Study the drawing (mm; zero at the part's minimum x, y, z) and answer. A direction names the side the tool comes from. Round coordinates to 2 decimals unless told otherwise and drop trailing zeros. Write each loop counter-clockwise with the first axis right and the second up, starting at its lowest first coordinate (ties: lowest second). Pieces come first, ordered by that corner, then holes. Notation, with made-up numbers: (-12, 81.5) - (30, 81.5) arc R23 cw to (30, 106.5) - close; hole circle Ø11 at (15, 2). An arc over 180 degrees is marked (long way). Return JSON: item names as keys, results as strings. Group by question number.
(1) Section A-A, the plane y = 2.5 is taken. Write down the section's boundary in (x, z), then the cut area to 3 significant figures.
(2) Which of the six approach directions +Z, -Z, +X, -X, +Y, -Y give full straight-line access (tool end or side, diameter ignored) to the marked faces 1, 2, 3 and 4?
(3) Each of these flat-tipped pins is pushed along its axis until it touches: pin 1 (1.2 mm diameter, centred on x = 4.5, z = 2, fed in from +Y); pin 2 (3.5 mm diameter, centred on x = 7.5, y = 8.5, fed in from -Z); pin 3 (3.5 mm diameter, centred on x = 9, z = 19, fed in from +Y); pin 4 (1.3 mm diameter, centred on x = 6, z = 13.5, fed in from +Y). Where does it stop, or does it pass through?
(4) Section D-D, the plane y = 28.5 is taken. Write down the section's boundary in (x, z).
(5) Section C-C, the plane x = 4.25 is taken. Write down the section's boundary in (y, z), then the cut area to 3 significant figures.
(6) Find the intervals of material crossed by line 1 along Y through (x, z) = (7, 2); line 2 along Z through (x, y) = (1, 17.5); line 3 along Y through (x, z) = (3.5, 25.5), in increasing order. Write a range as [from, to].
(7) Section B-B, the plane z = 23.5 is taken. Write down the section's boundary in (x, y).
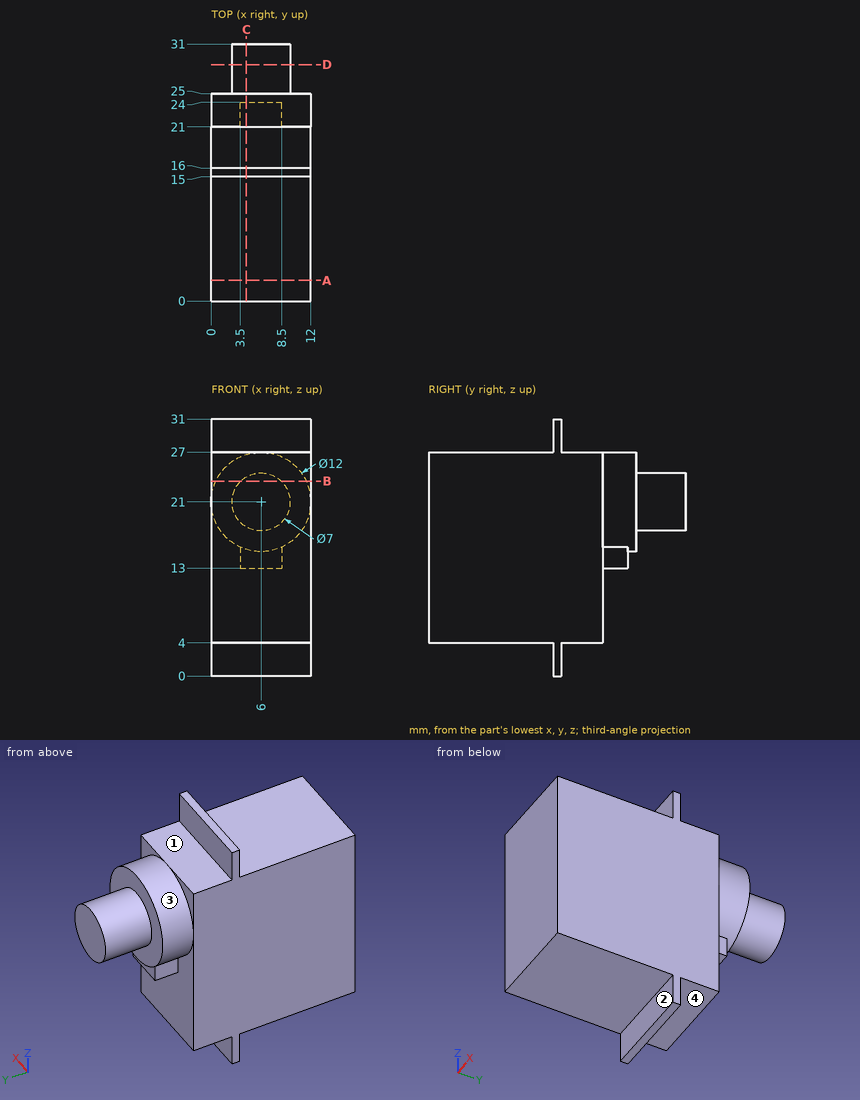
Working result:
{
 "1": {"outline": "(0, 4) - (12, 4) - (12, 27) - (0, 27) - close", "area": "276 mm^2"},
 "2": {"face 1": "+Z, +X, -X, +Y", "face 2": "-Z, +X, -X, -Y", "face 3": "+Y", "face 4": "-Z, +X, -X, +Y"},
 "3": {"pin 1": "stops at y = 16", "pin 2": "stops at z = 4", "pin 3": "stops at y = 31", "pin 4": "stops at y = 24"},
 "4": {"outline": "circle Ø7 at (6, 21)"},
 "5": {"outline": "(0, 4) - (15, 4) - (15, 0) - (16, 0) - (16, 4) - (21, 4) - (21, 13) - (24, 13) - (24, 15.26) - (25, 15.26) - (25, 17.97) - (31, 17.97) - (31, 24.03) - (25, 24.03) - (25, 26.74) - (21, 26.74) - (21, 27) - (16, 27) - (16, 31) - (15, 31) - (15, 27) - (0, 27) - close", "area": "580 mm^2"},
 "6": {"line 1": "y = [15, 16]", "line 2": "z = [4, 27]", "line 3": "y = [0, 25]"},
 "7": {"outline": "(0, 0) - (12, 0) - (12, 21) - (11.45, 21) - (11.45, 25) - (8.45, 25) - (8.45, 31) - (3.55, 31) - (3.55, 25) - (0.55, 25) - (0.55, 21) - (0, 21) - close"}
}
